```python
from build123d import *

# Parameters (mm, degrees)
F1_DEPTH = 12.7
F2_DEPTH = 101.6
F3_DEPTH = 76.2


with BuildPart() as f1:
    # F0 (on Top) → F1 (new body)
    with BuildSketch(Plane.XY):
        with BuildLine():
            ThreePointArc((-16.8005208253, -19.05), (-25.4, 0), (-16.8005208253, 19.05))
            Line((-16.8005208253, 19.05), (-63.5, 19.05))
            ThreePointArc((-63.5, 19.05), (-50.0296158184, 13.4703841816), (-44.45, 0))
            ThreePointArc((-44.45, 0), (-50.0296158184, -13.4703841816), (-63.5, -19.05))
            Line((-63.5, -19.05), (-16.8005208253, -19.05))
        make_face()
        with BuildLine():
            ThreePointArc((-82.55, 1.56e-07), (-76.9703841264, 13.4703842368), (-63.5, 19.05))
            Line((-63.5, 19.05), (-82.55, 19.05))
            Line((-82.55, 19.05), (-82.55, 1.56e-07))
        make_face()
        with BuildLine():
            Line((-82.55, -19.05), (-63.5, -19.05))
            ThreePointArc((-63.5, -19.05), (-76.9703842368, -13.4703841264), (-82.55, 1.56e-07))
            Line((-82.55, 1.56e-07), (-82.55, -19.05))
        make_face()
        with BuildLine():
            Line((82.55, 19.05), (63.5, 19.05))
            ThreePointArc((63.5, 19.05), (76.9703841816, 13.4703841816), (82.55, 0))
            Line((82.55, 0), (82.55, 19.05))
        make_face()
        with BuildLine():
            ThreePointArc((82.55, 0), (76.9703841816, -13.4703841816), (63.5, -19.05))
            Line((63.5, -19.05), (82.55, -19.05))
            Line((82.55, -19.05), (82.55, 0))
        make_face()
        with BuildLine():
            ThreePointArc((16.8005208253, 19.05), (23.1505208253, 10.4505208253), (25.4, 0))
            ThreePointArc((25.4, 0), (23.1505208253, -10.4505208253), (16.8005208253, -19.05))
            Line((16.8005208253, -19.05), (63.5, -19.05))
            ThreePointArc((63.5, -19.05), (44.45, 0), (63.5, 19.05))
            Line((63.5, 19.05), (16.8005208253, 19.05))
        make_face()
        with BuildLine():
            ThreePointArc((82.55, 0), (76.9703841816, 13.4703841816), (63.5, 19.05))
            ThreePointArc((63.5, 19.05), (44.45, 0), (63.5, -19.05))
            ThreePointArc((63.5, -19.05), (76.9703841816, -13.4703841816), (82.55, 0))
        make_face()
        with BuildLine():
            ThreePointArc((19.05, 0), (13.4703841605, 13.4703842027), (-5.96e-08, 19.05))
            ThreePointArc((-5.96e-08, 19.05), (-19.05, 7.1e-09), (-7.38e-08, -19.05))
            ThreePointArc((-7.38e-08, -19.05), (13.4703841555, -13.4703842077), (19.05, 0))
        make_face()
        with BuildLine():
            ThreePointArc((16.8005208253, -19.05), (23.1505208253, -10.4505208253), (25.4, 0))
            ThreePointArc((25.4, 0), (23.1505208253, 10.4505208253), (16.8005208253, 19.05))
            Line((16.8005208253, 19.05), (-5.96e-08, 19.05))
            ThreePointArc((-5.96e-08, 19.05), (13.4703841605, 13.4703842027), (19.05, 0))
            ThreePointArc((19.05, 0), (13.4703841555, -13.4703842077), (-7.38e-08, -19.05))
            Line((-7.38e-08, -19.05), (16.8005208253, -19.05))
        make_face()
        with BuildLine():
            Line((-5.96e-08, 19.05), (-16.8005208253, 19.05))
            ThreePointArc((-16.8005208253, 19.05), (-25.4, 0), (-16.8005208253, -19.05))
            Line((-16.8005208253, -19.05), (-7.38e-08, -19.05))
            ThreePointArc((-7.38e-08, -19.05), (-19.05, 7.1e-09), (-5.96e-08, 19.05))
        make_face()
        with BuildLine():
            ThreePointArc((-44.45, 0), (-50.0296158184, 13.4703841816), (-63.5, 19.05))
            ThreePointArc((-63.5, 19.05), (-76.9703841264, 13.4703842368), (-82.55, 1.56e-07))
            ThreePointArc((-82.55, 1.56e-07), (-76.9703842368, -13.4703841264), (-63.5, -19.05))
            ThreePointArc((-63.5, -19.05), (-50.0296158184, -13.4703841816), (-44.45, 0))
        make_face()
    extrude(amount=F1_DEPTH)

    # F0 (on Top) → F2 (join)
    with BuildSketch(Plane.XY):
        with BuildLine():
            Line((-5.96e-08, 19.05), (16.8005208253, 19.05))
            ThreePointArc((16.8005208253, 19.05), (0, 25.4), (-16.8005208253, 19.05))
            Line((-16.8005208253, 19.05), (-5.96e-08, 19.05))
        make_face()
        with BuildLine():
            ThreePointArc((16.8005208253, -19.05), (23.1505208253, -10.4505208253), (25.4, 0))
            ThreePointArc((25.4, 0), (23.1505208253, 10.4505208253), (16.8005208253, 19.05))
            Line((16.8005208253, 19.05), (-5.96e-08, 19.05))
            ThreePointArc((-5.96e-08, 19.05), (13.4703841605, 13.4703842027), (19.05, 0))
            ThreePointArc((19.05, 0), (13.4703841555, -13.4703842077), (-7.38e-08, -19.05))
            Line((-7.38e-08, -19.05), (16.8005208253, -19.05))
        make_face()
        with BuildLine():
            ThreePointArc((19.05, 0), (13.4703841605, 13.4703842027), (-5.96e-08, 19.05))
            ThreePointArc((-5.96e-08, 19.05), (-19.05, 7.1e-09), (-7.38e-08, -19.05))
            ThreePointArc((-7.38e-08, -19.05), (13.4703841555, -13.4703842077), (19.05, 0))
        make_face()
        with BuildLine():
            Line((-5.96e-08, 19.05), (-16.8005208253, 19.05))
            ThreePointArc((-16.8005208253, 19.05), (-25.4, 0), (-16.8005208253, -19.05))
            Line((-16.8005208253, -19.05), (-7.38e-08, -19.05))
            ThreePointArc((-7.38e-08, -19.05), (-19.05, 7.1e-09), (-5.96e-08, 19.05))
        make_face()
        with BuildLine():
            ThreePointArc((-16.8005208253, -19.05), (0, -25.4), (16.8005208253, -19.05))
            Line((16.8005208253, -19.05), (-7.38e-08, -19.05))
            Line((-7.38e-08, -19.05), (-16.8005208253, -19.05))
        make_face()
    extrude(amount=F2_DEPTH)

    # F0 (on Top) → F3 (join)
    with BuildSketch(Plane.XY):
        with BuildLine():
            ThreePointArc((82.55, 0), (76.9703841816, 13.4703841816), (63.5, 19.05))
            ThreePointArc((63.5, 19.05), (44.45, 0), (63.5, -19.05))
            ThreePointArc((63.5, -19.05), (76.9703841816, -13.4703841816), (82.55, 0))
        make_face()
        with BuildLine():
            ThreePointArc((19.05, 0), (13.4703841605, 13.4703842027), (-5.96e-08, 19.05))
            ThreePointArc((-5.96e-08, 19.05), (-19.05, 7.1e-09), (-7.38e-08, -19.05))
            ThreePointArc((-7.38e-08, -19.05), (13.4703841555, -13.4703842077), (19.05, 0))
        make_face()
        with BuildLine():
            ThreePointArc((-44.45, 0), (-50.0296158184, 13.4703841816), (-63.5, 19.05))
            ThreePointArc((-63.5, 19.05), (-76.9703841264, 13.4703842368), (-82.55, 1.56e-07))
            ThreePointArc((-82.55, 1.56e-07), (-76.9703842368, -13.4703841264), (-63.5, -19.05))
            ThreePointArc((-63.5, -19.05), (-50.0296158184, -13.4703841816), (-44.45, 0))
        make_face()
    extrude(amount=-F3_DEPTH)


solid = f1.part
```
Geometry: final body of the model. Coordinates: model frame, mm. A direction names the side the tool comes from. Round coordinates to 2 decimals unless told otherwise and drop trailing zeros. Write each loop counter-clockwise with the first axis right and the second up, starting at its lowest first coordinate (ties: lowest second). Pieces come first, ordered by that corner, then holes.
Item 1: Material intervals for L1, parallel to X at y = 7.5, z = -40.5; L2, parallel to X at y = -9, z = -43.5; L3, parallel to Z at x = -66, y = -12.5, sorted ascending.
Item 2: Pin query (flat end, axial travel): P1, Ø6, axis at x = 23.5, z = 73, coming from the -Y side; P2, Ø1, axis at x = 53.5, z = -49.5, coming from the -Y side; P3, Ø1, axis at x = 52.5, z = 2.5, coming from the -Y side. Return the tip coordinate at first contact, or that it passes through.
Item 3: Set-up query: faces 1 (the face through (50, 19.05, 6)), 2 (the face through (-79, 15, 0)), 3 (the face through (79, -15, 0)), 4 (the face through (44.47, 0.84, -37.57)). Return all of +Z, -Z, +X, -X, +Y, -Y with unobstructed straight access to the full face (end or side cutting, diameter ignored); none if empty.
Item 4: Mould query, pull axis Y, two halves, no side actions, for faces 5 (the face through (-49, 19.05, 6)), 6 (the face through (-50, -19.05, 6)), 7 (the face through (-4.13, -18.597, -37.567)), 8 (the face through (-79, -14, 0)). Classes: +Y half, -Y half, draft (parallel to the pull), parting line (faces both ways), or undercut.
Item 5: Section query A-A (z = -27.5). Return loops of the section in (x, y), plus the area to 3 significant figures.
Item 6: Section query B-B (y = 16). Return loops of the section in (x, z), plus the area to 3 significant figures.
Item 7: Section query D-D (y = -11). Return loops of the section in (x, z), plus the area to 3 significant figures.
Item 8: Section query C-C (x = 0). Return loops of the section in (y, z).
Completed:
1. L1: x = -81.01 to -45.99, -17.51 to 17.51, 45.99 to 81.01
1. L2: x = -80.29 to -46.71, -16.79 to 16.79, 46.71 to 80.29
1. L3: z = -76.2 to 12.7
2. P1: stops at y = -15
2. P2: stops at y = -16.51
2. P3: stops at y = -19.05
3. face 1: +Z, -Z, +X, +Y
3. face 2: -Z, -X, +Y
3. face 3: -Z, +X, -Y
3. face 4: -Z
4. face 5: +Y half
4. face 6: -Y half
4. face 7: parting line
4. face 8: draft
5. outline: circle Ø38.1 at (-63.5, 0); circle Ø38.1 at (0, 0); circle Ø38.1 at (63.5, 0)
5. area: 3,420 mm2
6. outline: (-82.55, 0) - (-73.84, 0) - (-73.84, -76.2) - (-53.16, -76.2) - (-53.16, 0) - (-10.34, 0) - (-10.34, -76.2) - (10.34, -76.2) - (10.34, 0) - (53.16, 0) - (53.16, -76.2) - (73.84, -76.2) - (73.84, 0) - (82.55, 0) - (82.55, 12.7) - (19.73, 12.7) - (19.73, 101.6) - (-19.73, 101.6) - (-19.73, 12.7) - (-82.55, 12.7) - close
6. area: 10,300 mm2
7. outline: (-82.55, 0) - (-79.05, 0) - (-79.05, -76.2) - (-47.95, -76.2) - (-47.95, 0) - (-15.55, 0) - (-15.55, -76.2) - (15.55, -76.2) - (15.55, 0) - (47.95, 0) - (47.95, -76.2) - (79.05, -76.2) - (79.05, 0) - (82.55, 0) - (82.55, 12.7) - (22.89, 12.7) - (22.89, 101.6) - (-22.89, 101.6) - (-22.89, 12.7) - (-82.55, 12.7) - close
7. area: 13,300 mm2
8. outline: (-25.4, 0) - (-19.05, 0) - (-19.05, -76.2) - (19.05, -76.2) - (19.05, 0) - (25.4, 0) - (25.4, 101.6) - (-25.4, 101.6) - close
